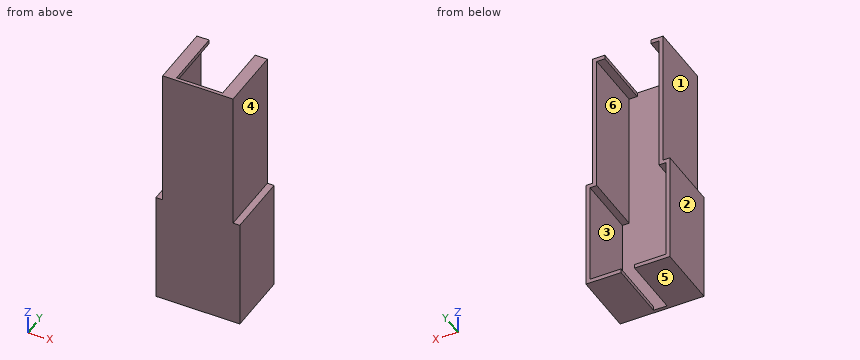
from build123d import *

# Parameters (mm, degrees)
SKETCH1_W           = 52
SKETCH1_H           = 103
SKETCH1_W_2         = 62
SKETCH1_H_2         = 82
BOSS_EXTRUDE1_DEPTH = 2.5
SKETCH2_W           = 3
SKETCH2_H           = 100
SKETCH2_H_2         = 76
SKETCH2_W_2         = 2
SKETCH2_H_3         = 3
SKETCH2_W_3         = 56
SKETCH2_W_4         = 46
BOSS_EXTRUDE2_DEPTH = 45
SKETCH4_W           = 10
SKETCH4_H           = 3
SKETCH4_W_2         = 34
CUT_EXTRUDE1_DEPTH  = 45


with BuildPart() as part:
    # Sketch1 → Boss-Extrude1 (new body)
    with BuildSketch(Plane(origin=(0, 0, 0), x_dir=(1, 0, 0), z_dir=(0, 1, 0))):
        with Locations((0.405405405, -109.013513514)):
            Rectangle(SKETCH1_W, SKETCH1_H)
        with Locations((0.405405405, -16.513513514)):
            Rectangle(SKETCH1_W_2, SKETCH1_H_2)
    extrude(amount=BOSS_EXTRUDE1_DEPTH)

    # Sketch2 → Boss-Extrude2 (add)
    with BuildSketch(Plane(origin=(0, 2.5, 0), x_dir=(1, 0, 0), z_dir=(0, 1, 0))):
        with Locations((-24.094594595, -107.513513514)):
            Rectangle(SKETCH2_W, SKETCH2_H)
        with Locations((24.905405405, -107.513513514)):
            Rectangle(SKETCH2_W, SKETCH2_H)
        with Locations((29.905405405, -16.513513514)):
            Rectangle(SKETCH2_W, SKETCH2_H_2)
        with Locations((-29.094594595, -16.513513514)):
            Rectangle(SKETCH2_W, SKETCH2_H_2)
        with Locations((-26.594594595, -56.013513514)):
            Rectangle(SKETCH2_W_2, SKETCH2_H_3)
        with Locations((-24.094594595, -56.013513514)):
            Rectangle(SKETCH2_W, SKETCH2_H_3)
        with Locations((-29.094594595, -56.013513514)):
            Rectangle(SKETCH2_W, SKETCH2_H_3)
        with Locations((29.905405405, -56.013513514)):
            Rectangle(SKETCH2_W, SKETCH2_H_3)
        with Locations((27.405405405, -56.013513514)):
            Rectangle(SKETCH2_W_2, SKETCH2_H_3)
        with Locations((24.905405405, -56.013513514)):
            Rectangle(SKETCH2_W, SKETCH2_H_3)
        with Locations((-29.094594595, 22.986486486)):
            Rectangle(SKETCH2_W, SKETCH2_H_3)
        with Locations((29.905405405, 22.986486486)):
            Rectangle(SKETCH2_W, SKETCH2_H_3)
        with Locations((0.405405405, 22.986486486)):
            Rectangle(SKETCH2_W_3, SKETCH2_H_3)
        with Locations((-24.094594595, -159.013513514)):
            Rectangle(SKETCH2_W, SKETCH2_H_3)
        with Locations((0.405405405, -159.013513514)):
            Rectangle(SKETCH2_W_4, SKETCH2_H_3)
        with Locations((24.905405405, -159.013513514)):
            Rectangle(SKETCH2_W, SKETCH2_H_3)
    extrude(amount=BOSS_EXTRUDE2_DEPTH)

    # Sketch4 → Cut-Extrude1 (cut)
    with BuildSketch(Plane(origin=(0, 47.5, 0), x_dir=(1, 0, 0), z_dir=(0, 1, 0))):
        with Locations((0.405405405, 22.986486486)):
            Rectangle(SKETCH4_W, SKETCH4_H)
        with Locations((0.405405405, -159.013513514)):
            Rectangle(SKETCH4_W_2, SKETCH4_H)
    extrude(amount=-CUT_EXTRUDE1_DEPTH, mode=Mode.SUBTRACT)


solid = part.part
Part model, mm, in its own coordinate system. Face numbers are marked on the shaded views. A direction names the side the tool comes from. Coordinates: 2 decimals unless noted, no trailing zeros. Write each loop counter-clockwise with the first axis right and the second up, starting at its lowest first coordinate (ties: lowest second). Pieces come first, ordered by that corner, then holes. Notation, with made-up numbers: (73.5, 28.5) - (82.5, 28.5) arc R15 ccw to (82.5, 51.5) - close; hole circle Ø8 at (-20, -21). An arc over 180 degrees is marked (long way). Put each result on its own line as item: value.
1. Band-saw the part on A-A (y = 21). Write the cut outline in (x, z).
Final values:
outline: (-30.59, -24.49) - (-4.59, -24.49) - (-4.59, -21.49) - (-27.59, -21.49) - (-27.59, 54.51) - (-22.59, 54.51) - (-22.59, 157.51) - (-16.59, 157.51) - (-16.59, 160.51) - (-25.59, 160.51) - (-25.59, 57.51) - (-30.59, 57.51) - close; (5.41, -24.49) - (31.41, -24.49) - (31.41, 57.51) - (26.41, 57.51) - (26.41, 160.51) - (17.41, 160.51) - (17.41, 157.51) - (23.41, 157.51) - (23.41, 54.51) - (28.41, 54.51) - (28.41, -21.49) - (5.41, -21.49) - close
2. Band-saw the part on B-B (z = 23). Write the cut outline in (x, y).
Final values:
outline: (-30.59, 0) - (31.41, 0) - (31.41, 47.5) - (28.41, 47.5) - (28.41, 2.5) - (-27.59, 2.5) - (-27.59, 47.5) - (-30.59, 47.5) - close
3. Band-saw the part on C-C (x = -9). Write the cut outline in (y, z).
Final values:
outline: (0, -24.49) - (47.5, -24.49) - (47.5, -21.49) - (2.5, -21.49) - (2.5, 160.51) - (0, 160.51) - close
4. Band-saw the part on D-D (z = 129). Write the cut outline in (x, y).
Final values:
outline: (-25.59, 0) - (26.41, 0) - (26.41, 47.5) - (23.41, 47.5) - (23.41, 2.5) - (-22.59, 2.5) - (-22.59, 47.5) - (-25.59, 47.5) - close
5. 3-axis set-ups, long thin cutter, end or side, ignore diameter. For the marked faces 1, 2 and 3: which of +Z, -Z, +X, -X, +Y, -Y reach the whole face in a straight line?
Final values:
face 1: +Z, -X, +Y, -Y
face 2: +Z, -Z, -X, +Y, -Y
face 3: +Y
6. Probe line 1 along X through (y, z) = (24.5, 15.5); line 2 along Z through (x, y) = (-21, 38); line 3 along X through (y, z) = (15.5, 78.5). List the from-to ranges inside material, lowest first. Write a range as [from, to].
Final values:
line 1: x = [-30.59, -27.59], [28.41, 31.41]
line 2: z = [-24.49, -21.49], [157.51, 160.51]
line 3: x = [-25.59, -22.59], [23.41, 26.41]
7. Flat gauge pins, fed straight in: pin 1 Ø3.5 at (y, z) = (18, 158.5) entering from -X; pin 2 Ø13.5 at (y, z) = (35, 92) entering from +X; pin 3 Ø18.5 at (x, y) = (-16, 19.5) entering from +Z; pin 4 Ø2.5 at (x, y) = (-29, 16.5) entering from +Z. Where does each tip first touch, or does it go through?
Final values:
pin 1: stops at x = -25.59
pin 2: stops at x = 26.41
pin 3: stops at z = 160.51
pin 4: stops at z = 57.51
8. Two-plate mould, pull along Z, no slides. Class the marked faces 4, 5 and 6: +Z half, -Z half, draft (parallel to the pull), parting line (faces both ways), or undercut.
Final values:
face 4: draft
face 5: -Z half
face 6: undercut
